```python
from build123d import *

# Parameters (mm, degrees)
SKETCH1_R           = 20.32
SKETCH1_R_2         = 4.6355
BOSS_EXTRUDE1_DEPTH = 10
SKETCH2_R           = 16.51
SKETCH2_R_2         = 11.43
BOSS_EXTRUDE2_DEPTH = 19.05
BOSS_EXTRUDE3_START = 10.16
SKETCH3_R           = 20.32
SKETCH3_R_2         = 4.6355
BOSS_EXTRUDE3_DEPTH = 10.16
CUT_EXTRUDE1_START  = -12
SKETCH4_R           = 11.43
CUT_EXTRUDE1_DEPTH  = 12
SKETCH5_R           = 8.5
CUT_EXTRUDE2_DEPTH  = 1.5


with BuildPart() as part:
    # Sketch1 → Boss-Extrude1 (new body)
    with BuildSketch(Plane(origin=(0, 0, 0), x_dir=(1, 0, 0), z_dir=(0, 1, 0))):
        with Locations(Location((0, 0, 0), (0, 0, 270))):
            Circle(SKETCH1_R)
        with Locations(Location((0, 0, 0), (0, 0, 270))):
            Circle(SKETCH1_R_2, mode=Mode.SUBTRACT)
    extrude(amount=BOSS_EXTRUDE1_DEPTH)

    # Sketch2 → Boss-Extrude2 (add)
    with BuildSketch(Plane(origin=(0, 10, 0), x_dir=(1, 0, 0), z_dir=(0, 1, 0))):
        with Locations(Location((0, 0, 0), (0, 0, 90))):
            Circle(SKETCH2_R)
        with Locations(Location((0, 0, 0), (0, 0, 90))):
            Circle(SKETCH2_R_2, mode=Mode.SUBTRACT)
    extrude(amount=BOSS_EXTRUDE2_DEPTH)

    # Sketch3 → Boss-Extrude3 (add)
    with BuildSketch(Plane(origin=(0, 0, 0), x_dir=(-1, 0, 0), z_dir=(0, -1, 0)).offset(BOSS_EXTRUDE3_START)):
        with Locations(Location((0, 0, 0), (0, 0, 90))):
            Circle(SKETCH3_R)
        with Locations(Location((0, 0, 0), (0, 0, 90))):
            Circle(SKETCH3_R_2, mode=Mode.SUBTRACT)
    extrude(amount=-BOSS_EXTRUDE3_DEPTH)

    # Sketch4 → Cut-Extrude1 (cut)
    with BuildSketch(Plane(origin=(0, 10, 0), x_dir=(1, 0, 0), z_dir=(0, 1, 0)).offset(CUT_EXTRUDE1_START)):
        with Locations(Location((0, 0, 0), (0, 0, 90))):
            Circle(SKETCH4_R)
    extrude(amount=CUT_EXTRUDE1_DEPTH, mode=Mode.SUBTRACT)

    # Sketch5 → Cut-Extrude2 (cut)
    with BuildSketch(Plane(origin=(0, -2, 0), x_dir=(1, 0, 0), z_dir=(0, 1, 0))):
        with Locations(Location((0, 0, 0), (0, 0, 270))):
            Circle(SKETCH5_R)
    extrude(amount=-CUT_EXTRUDE2_DEPTH, mode=Mode.SUBTRACT)


solid = part.part
```
Input: part model. Units: mm. Frame: model coordinates. A direction names the side the tool comes from. Give positions to 0.01 mm unless a question says otherwise; leave off trailing zeros. Order: outer loops, then holes, each group sorted by start corner. A loop starts at its lowest first (then second) coordinate and runs counter-clockwise, first axis right, second up. Notation, with made-up numbers: M -13.75,13 L 1.25,13 A15 cw 1.25,32 Z; hole C -24,46.25 d8. An arc over 180 degrees is marked long. One line per question, with ' | ' between items.
1) Section D-D on z = 10.5. Output: boundary loops of the cut face in (x, y), and give its area (3 significant figures).
Filled in:
outline: M -17.4,-10.16 L 17.4,-10.16 L 17.4,10 L 12.74,10 L 12.74,29.05 L 4.52,29.05 L 4.52,-2 L -4.52,-2 L -4.52,29.05 L -12.74,29.05 L -12.74,10 L -17.4,10 Z | area: 906 mm2
2) Draft query along Z for faces 3 (the face through (10.05, 19.39, 13.1)), 4 (the face through (17, 10, 0)), 5 (the face through (-9, -2, 0)). Return one class per face: pulls with the +Z half, pulls with the -Z half, needs draft (parallel to the pull), parting line crosses it, or undercut.
Filled in:
face 3: parting line crosses it | face 4: needs draft | face 5: undercut
3) Access query for faces 1 (the face through (-4, -3.5, 4)), 2 (the face through (5, -10.16, 0)). Directions: +Z, -Z, +X, -X, +Y, -Y. A direction counts if a zero-diameter tool reaches every point of the face in a straight line with its end or side. Return the directions, or none.
Filled in:
face 1: +Y | face 2: +Z, -Z, +X, -X, -Y
4) Section A-A on x = 0. Output: boundary loops of the cut face in (y, z).
Filled in:
outline: M -10.16,-20.32 L 10,-20.32 L 10,-16.51 L 29.05,-16.51 L 29.05,-11.43 L -2,-11.43 L -2,-8.5 L -3.5,-8.5 L -3.5,-4.64 L -10.16,-4.64 Z; M -10.16,4.64 L -3.5,4.64 L -3.5,8.5 L -2,8.5 L -2,11.43 L 29.05,11.43 L 29.05,16.51 L 10,16.51 L 10,20.32 L -10.16,20.32 Z
5) Ray query, L1, parallel to X at y = 6, z = 0; L2, parallel to X at y = -7, z = 0; L3, parallel to Z at x = -0.5, y = 26. Return the intervals inside material, ascending.
Filled in:
L1: x = -20.32 to -11.43, 11.43 to 20.32 | L2: x = -20.32 to -4.64, 4.64 to 20.32 | L3: z = -16.5 to -11.42, 11.42 to 16.5
6) Section B-B on z = -4. Output: boundary loops of the cut face in (x, y).
Filled in:
outline: M -19.92,-10.16 L -2.34,-10.16 L -2.34,-3.5 L -7.5,-3.5 L -7.5,-2 L -10.71,-2 L -10.71,29.05 L -16.02,29.05 L -16.02,10 L -19.92,10 Z; M 2.34,-10.16 L 19.92,-10.16 L 19.92,10 L 16.02,10 L 16.02,29.05 L 10.71,29.05 L 10.71,-2 L 7.5,-2 L 7.5,-3.5 L 2.34,-3.5 Z
7) Contact query for flat-ended pins moving along their axis: P1, Ø13.5, axis at x = 0, z = 0, coming from the +Y side; P2, Ø10, axis at y = 0, z = 9.5, coming from the +X side; P3, Ø8.5, axis at x = 0, z = 0, coming from the +Y side; P4, Ø6, axis at y = 19.5, z = -12.5, coming from the +X side. Output: stop coordinate, or through.
Filled in:
P1: stops at y = -3.5 | P2: stops at x = 19.82 | P3: passes through | P4: stops at x = 13.5
8) Section C-C on y = 15.5. Output: boundary loops of the cut face in (x, z).
Filled in:
outline: C 0,0 d33.02; hole C 0,0 d22.86
